Check sheet for the drawn part. Datum: minimum x, y, z corner. Units: mm. A direction names the side the tool comes from. Give positions to 0.01 mm unless a question says otherwise; leave off trailing zeros. Loops run counter-clockwise (first coordinate to the right, second up) from the corner with the lowest first, then second, coordinate; pieces in that order, holes last.
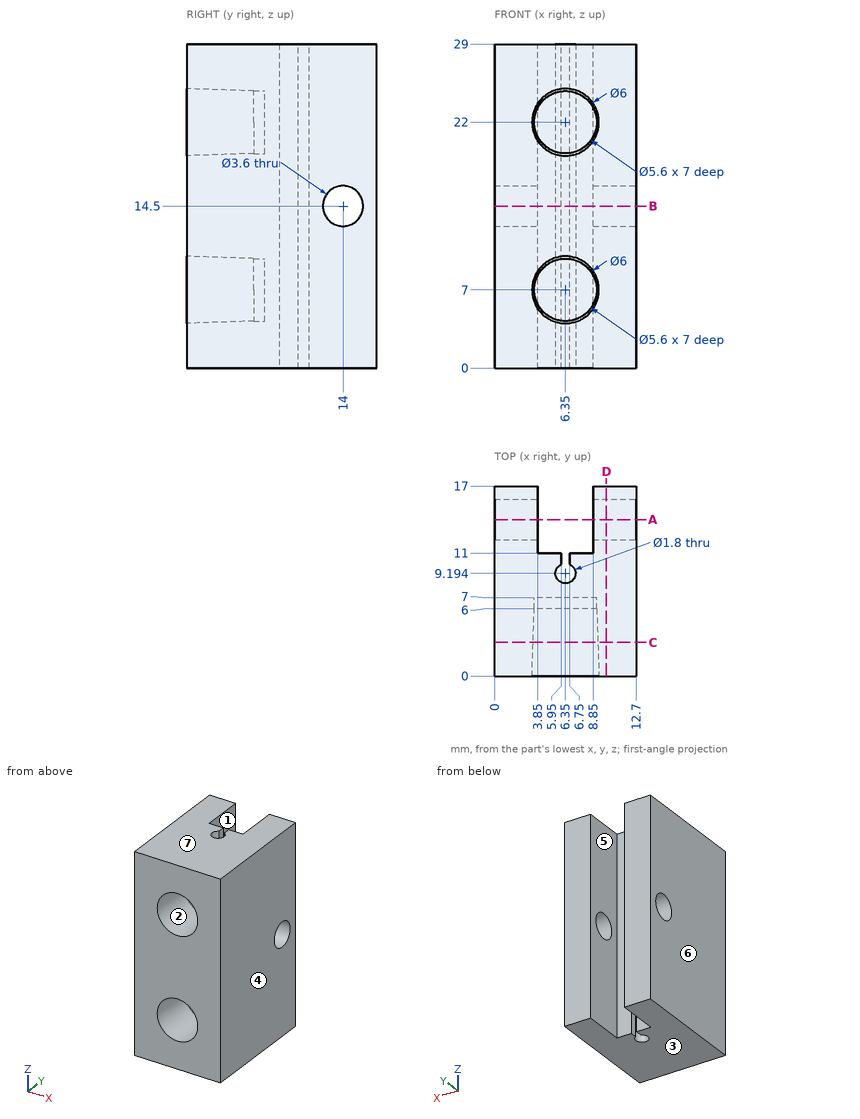
1) Sectioned sample at A-A on y = 14. Enter the section's corners in (x, z).
2) Mould release check, pull along X, two halves, no side actions. Record for the marked faces 4, 5, 6 and 7: +X half, -X half, draft (parallel to the pull), parting line (faces both ways), or undercut.
3) Tool access check on the marked faces 1, 2 and 3. Record the directions out of +Z, -Z, +X, -X, +Y, -Y that give a thin tool (end or side, any length) a straight path to the whole face; none if there is none.
4) Sectioned sample at D-D on x = 10. Enter the section's corners in (y, z), plus the area to 3 significant figures.
5) Sectioned sample at C-C on y = 3. Enter the section's corners in (x, z).
6) Depth check by flat-ended pin: P1, Ø2.5, axis at x = 6.35, y = 9.19, coming from the +Z side; P2, Ø1.7, axis at x = 5, z = 8, coming from the -Y side; P3, Ø0.6, axis at x = 4.5, z = 14.5, coming from the +Y side. Enter the tip coordinate at first touch or a pass-through.
7) Sectioned sample at B-B on z = 14.5. Enter the section's corners in (x, y).
8) Scan lines: line 1 along Z through (x, y) = (6.35, 6.35); line 2 along Y through (x, z) = (11.25, 14.5); line 3 along X through (y, z) = (6.7, 22). Record each from-to range of solid material in increasing order.
Determined:
1. outline: (0, 0) - (3.85, 0) - (3.85, 12.7) - (0, 12.7) - close; (0, 16.3) - (3.85, 16.3) - (3.85, 29) - (0, 29) - close; (8.85, 0) - (12.7, 0) - (12.7, 12.7) - (8.85, 12.7) - close; (8.85, 16.3) - (12.7, 16.3) - (12.7, 29) - (8.85, 29) - close
2. face 4: +X half
2. face 5: undercut
2. face 6: -X half
2. face 7: draft
3. face 1: +Z, -Z, +Y
3. face 2: -Y
3. face 3: -Z, +X, -X, +Y, -Y
4. outline: (0, 0) - (17, 0) - (17, 29) - (0, 29) - close; hole circle Ø3.6 at (14, 14.5)
4. area: 483 mm2
5. outline: (0, 0) - (12.7, 0) - (12.7, 29) - (0, 29) - close; hole circle Ø5.8 at (6.35, 7); hole circle Ø5.8 at (6.35, 22)
6. P1: stops at z = 29
6. P2: stops at y = 7
6. P3: stops at y = 11
7. outline: (0, 0) - (12.7, 0) - (12.7, 12.2) - (8.85, 12.2) - (8.85, 11) - (6.75, 11) - (6.75, 10) arc R0.9 cw (long way) to (5.95, 10) - (5.95, 11) - (3.85, 11) - (3.85, 12.2) - (0, 12.2) - close; (0, 15.8) - (3.85, 15.8) - (3.85, 17) - (0, 17) - close; (8.85, 15.8) - (12.7, 15.8) - (12.7, 17) - (8.85, 17) - close
8. line 1: z = 0 to 4.2, 9.8 to 19.2, 24.8 to 29
8. line 2: y = 0 to 12.2, 15.8 to 17
8. line 3: x = 0 to 3.55, 9.15 to 12.7
